Could you check a few things on this drawing? It's one solid part, dimensions in mm from its lowest x, y, z. A direction names the side the tool comes from. Round coordinates to 2 decimals unless told otherwise and drop trailing zeros. Loops run counter-clockwise (first coordinate to the right, second up) from the corner with the lowest first, then second, coordinate; pieces in that order, holes last. Notation, with made-up numbers: M 61,-1.75 L 115,-1.75 A24 cw 115,15.25 Z; hole C 12.25,-34.75 d5. An arc over 180 degrees is marked long. Return JSON: item names as keys, results as strings.
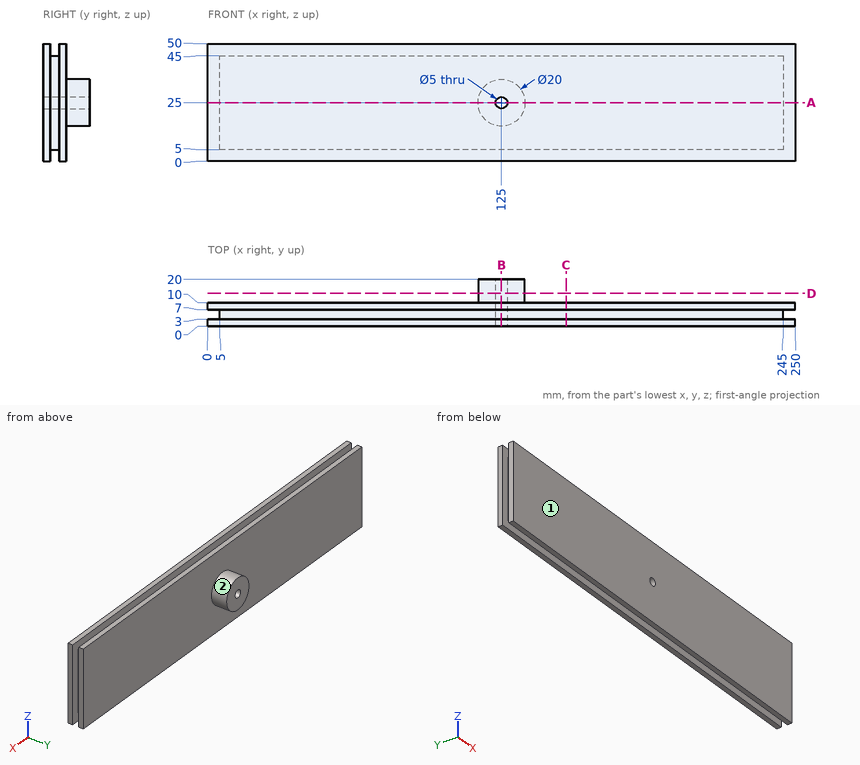
Q1. If I drill on line 1 along X through (y, z) = (9, 25); line 2 along X through (y, z) = (11, 25); line 3 along Z through (x, y) = (125, 5), over which ranges is the centre line in solid material (lowest first)?
Results:
{"line 1": "x = 0 to 122.5, 127.5 to 250", "line 2": "x = 115 to 122.5, 127.5 to 135", "line 3": "z = 5 to 22.5, 27.5 to 45"}
Q2. Suppose I cut it at A-A, the plane z = 25. Please give me the cut outline in (x, y).
Results:
{"outline": "M 0,0 L 122.5,0 L 122.5,20 L 115,20 L 115,10 L 0,10 L 0,7 L 5,7 L 5,3 L 0,3 Z; M 127.5,0 L 250,0 L 250,3 L 245,3 L 245,7 L 250,7 L 250,10 L 135,10 L 135,20 L 127.5,20 Z"}
Q3. Suppose I cut it at D-D, the plane y = 14. Please give me the cut outline in (x, z), plus the area to 3 significant figures.
Results:
{"outline": "C 125,25 d20; hole C 125,25 d5", "area": "295 mm2"}
Q4. Suppose I cut it at B-B, the plane x = 125. Please give me the cut outline in (y, z), plus the area to 3 significant figures.
Results:
{"outline": "M 0,0 L 3,0 L 3,5 L 7,5 L 7,0 L 10,0 L 10,15 L 20,15 L 20,22.5 L 0,22.5 Z; M 0,27.5 L 20,27.5 L 20,35 L 10,35 L 10,50 L 7,50 L 7,45 L 3,45 L 3,50 L 0,50 Z", "area": "560 mm2"}
Q5. On a 3-axis mill with a long thin cutter (end or side, diameter ignored), from which of +Z, -Z, +X, -X, +Y, -Y can I reach the whole of each face in a straight line? I mean the marked faces 1 and 2. Say none if no direction works.
Results:
{"face 1": "+Z, -Z, +X, -X, -Y", "face 2": "+Y"}
Q6. I'm going to push flat-ended pins straight in: pin 1 Ø1.5 at (y, z) = (4.5, 6.5) entering from -X; pin 2 Ø1.2 at (y, z) = (5, 29.5) entering from +X; pin 3 Ø1.2 at (x, y) = (152.5, 4) entering from +Z. Where does each tip first touch, or does it pass through?
Results:
{"pin 1": "stops at x = 5", "pin 2": "stops at x = 245", "pin 3": "stops at z = 45"}
Q7. Suppose I cut it at C-C, the plane x = 152.5. Please give me the cut outline in (y, z).
Results:
{"outline": "M 0,0 L 3,0 L 3,5 L 7,5 L 7,0 L 10,0 L 10,50 L 7,50 L 7,45 L 3,45 L 3,50 L 0,50 Z"}
